Autodesk Inventor part; units mm, degrees
ref_plane "YZ Plane" through (0, 0, 0) normal (1, 0, 0) x (0, 1, 0)
ref_plane "XZ Plane" through (0, 0, 0) normal (0, 1, 0) x (-1, 0, 0)
ref_plane "XY Plane" through (0, 0, 0) normal (0, 0, 1) x (1, 0, 0)
sketch "Sketch1" plane through (0, 0, 0) normal (0, 0, 1) x (1, 0, 0)
  line L0 (0, 0) -> (3.175, 0)
  line L1 (3.175, 0) -> (3.175, 38.1)
  line L2 (3.175, 38.1) -> (0, 38.1)
  line L3 (0, 38.1) -> (0, 0)
  line L4 (0, 0) -> (38.1, 0)
  line L5 (38.1, 0) -> (38.1, 3.175)
  line L6 (38.1, 3.175) -> (0, 3.175)
  line L7 (0, 3.175) -> (0, 0)
  line L8 (38.1, 0) -> (34.925, 0)
  line L9 (34.925, 0) -> (34.925, 38.1)
  line L10 (34.925, 38.1) -> (38.1, 38.1)
  line L11 (38.1, 38.1) -> (38.1, 0)
  dimension "d0" = 3.175
  dimension "d1" = 38.1
  dimension "d2" = 38.1
  dimension "d3" = 3.175
  dimension "d4" = 3.175
  dimension "d5" = 38.1
extrude "Extrusion1" add sketch "Sketch1" along normal blind 101.6
sketch "Sketch2" plane through (38.1, 0, 0) normal (1, 0, 0) x (0, 0, -1)
  line L0 (-101.6, 3.175) -> (0, 3.175)
  line L1 (0, 0) -> (0, 38.1)
  point P0 (-7.9375, 9.525)
  dimension "d8" = 6.35
  dimension "d9" = 7.9375
hole "Hole1" at (38.1, 9.525, 7.9375) direction (-1, 0, 0) diameter 6.35 end through all
sketch "Sketch3" plane through (38.1, 0, 0) normal (1, 0, 0) x (0, 0, -1)
  line L0 (0, 38.1) -> (-101.6, 38.1)
  line L1 (0, 0) -> (0, 38.1)
  point P0 (-22.225, 31.75)
  dimension "d17" = 6.35
  dimension "d18" = 22.225
hole "Hole2" at (38.1, 31.75, 22.225) direction (-1, 0, 0) diameter 6.35 end through all
ref_plane "Work Plane1" through (19.05, 3.175, 0) normal (-1, 0, 0) x (0, 0, 1)
fillet "Fillet1" radius 12.7 1 edges at (19.05, 0, 0)
sketch "Sketch4" plane through (0, 0, 101.6) normal (-1, 0, 0) x (0, 0, 1)
  line L0 (-78.4449, 41.9138) -> (31.1063, -12.1864)
  line L1 (31.1063, -12.1864) -> (58.2522, 42.7832)
  line L2 (58.2522, 42.7832) -> (-51.299, 96.8833)
  line L3 (-51.299, 96.8833) -> (-78.4449, 41.9138)
  arc A0 (-101.6, 12.7) -> (-88.9, 0) centre (-88.9, 12.7) ccw
  line L4 (-88.9, 0) -> (0, 0)
  line L5 (0, 38.1) -> (0, 0)
  line L6 (-101.6, 38.1) -> (0, 38.1)
  line L7 (-101.6, 38.1) -> (-101.6, 12.7)
  circle A1 centre (-79.375, 31.75) radius 3.175
  circle A2 centre (-93.6625, 9.525) radius 3.175
  line L8 (-97.3003, 3.175) -> (0, 3.175)
  point P0 (-101.6, 0)
  dimension "d27" = 9.525
  dimension "d28" = 6.35
extrude "Extrusion2" cut sketch "Sketch4" against normal through all contours L5 L6 L0 L3 L2 L1 | L0 L6 L5
fillet "Fillet2" radius 15.875 2 edges at (1.5875, 38.1, 0) (36.5125, 38.1, 0)
sketch "Sketch5" plane through (0, 0, 101.6) normal (0, -1, 0) x (1, 0, 0)
  line L0 (0, -88.9) -> (0, 0)
  point P0 (0, -101.6)
  point P1 (19.05, -25.4)
  dimension "d32" = 19.05
  dimension "d40" = 76.2
hole "Hole3" at (19.05, 0, 76.2) direction (0, 1, 0) diameter 6.35 end through all
sketch "Sketch6" plane through (0, 0, 101.6) normal (0, -1, 0) x (1, 0, 0)
  circle A0 centre (19.05, -25.4) radius 3.175
  circle A1 centre (19.05, -25.4) radius 3.175
  line L0 (38.1, -88.9) -> (0, -88.9)
  line L1 (38.1, -88.9) -> (38.1, 0)
  line L2 (0, 0) -> (38.1, 0)
  line L3 (0, -88.9) -> (0, 0)
  line L4 (-11.1164, -15.875) -> (47.1756, -15.875)
  line L5 (47.1756, -15.875) -> (47.1756, 8.1032)
  line L6 (47.1756, 8.1032) -> (-11.1164, 8.1032)
  line L7 (-11.1164, 8.1032) -> (-11.1164, -15.875)
  point P0 (0, -101.6)
  dimension "d41" = 9.525
  dimension "d42" = 6.35
extrude "Extrusion3" cut sketch "Sketch6" against normal through all contours L4 L3 L2 L1 | L1 L2 L3 L4 L7 L6 L5
fillet "Fillet3" radius 19.05 2 edges at (0, 5.5073, 85.725) (38.1, 5.5073, 85.725)
sketch "Sketch7" plane through (0, 0, 12.7) normal (0, -1, 0) x (1, 0, 0)
  circle A0 centre (19.05, 63.5) radius 3.175
  line L0 (19.05, 63.5) -> (19.05, 60.325) construction
  line L1 (15.875, 63.5) -> (15.875, 60.325)
  line L2 (22.225, 60.325) -> (22.225, 63.5)
  arc A1 (22.225, 63.5) -> (15.875, 63.5) centre (19.05, 63.5) ccw
  arc A2 (15.875, 60.325) -> (22.225, 60.325) centre (19.05, 60.325) ccw
  point P0 (0, -12.7)
  point P1 (19.05, 61.9125)
  dimension "d46" = 3.175
extrude "Extrusion4" cut sketch "Sketch7" against normal blind 25.4 contours L2 A2 L1 A0
properties part number "CAR_048_NewCarouselTensioner1.5UChannel" material "Aluminum 6061"
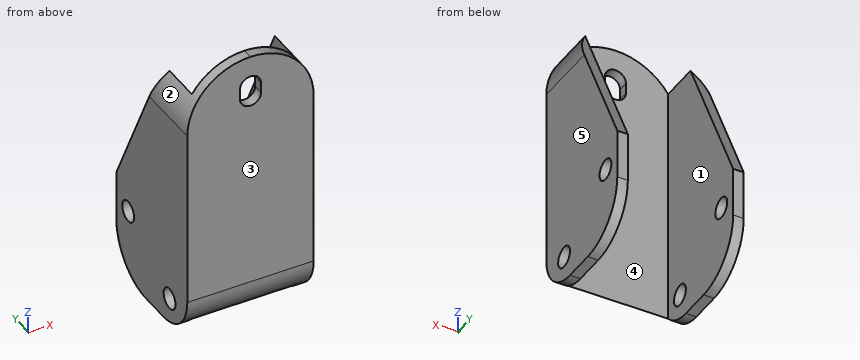
Part model, mm, in its own coordinate system. Face numbers are marked on the shaded views. A direction names the side the tool comes from. Give positions to 0.01 mm unless a question says otherwise; leave off trailing zeros. Write each loop counter-clockwise with the first axis right and the second up, starting at its lowest first coordinate (ties: lowest second). Pieces come first, ordered by that corner, then holes. Notation, with made-up numbers: (62.25, -16.5) -> (87.25, -16.5) arc R23 cw to (87.25, 17.5) -> close; hole circle Ø4 at (62, 78.5). An arc over 180 degrees is marked (long way). Put each result on its own line as item: value. Start each with the question number.
Item 1: Wall check: L1, parallel to X at y = 20.5, z = 54 (3 decimals); L2, parallel to Y at x = 13, z = 60 (3 decimals); L3, parallel to Z at x = 16.5, y = 2.5. Give the ranges that are in metal, low to high. Write a range as [from, to].
Item 2: Which spindle directions (+Z, -Z, +X, -X, +Y, -Y) get a long thin tool onto all of the face, cutting with end or side? Do the marked faces 4 and 5. Say none if no direction does.
Item 3: Pin check, flat tips, straight feed: pin 1 Ø3 at (x, z) = (26, 69.5) entering from +Y (3 decimals); pin 2 Ø6 at (y, z) = (29.5, 60) entering from -X; pin 3 Ø2.5 at (y, z) = (1.5, 75) entering from -X; pin 4 Ø1 at (x, z) = (17.5, 9) entering from -Y. Stop position of each tip, or through.
Item 4: Pull direction X, two halves, no side cores. Call the marked faces 1, 2 and 3: pulls with the +X half, pulls with the -X half, needs draft (parallel to the pull), parting line crosses it, or undercut.
Item 5: Cut at A-A (y = 16.5). List the corners of the cut face in (x, z) (3 decimals), then the cut area to 3 significant figures.
Item 6: Cut at D-D (x = 14). List the corners of the cut face in (y, z) (3 decimals).
Item 7: Cut at B-B (y = 31.75). List the corners of the cut face in (x, z) (3 decimals).
Item 8: Cut at C-C (z = 65.5). List the corners of the cut face in (x, y) (3 decimals), then the cut area to 3 significant figures.
Answer list:
1. L1: x = [0, 3.175], [34.925, 38.1]
1. L2: y = [0, 3.175]
1. L3: z = [5.13, 71.13], [78.09, 85.55]
2. face 4: +Z, -Z, +Y
2. face 5: +Z, -Z, +X, +Y, -Y
3. pin 1: stops at y = 3.175
3. pin 2: passes through
3. pin 3: stops at x = 1.36
3. pin 4: stops at y = 0.41
4. face 1: undercut
4. face 2: pulls with the -X half
4. face 3: needs draft
5. outline: (0, 0) -> (3.175, 0) -> (3.175, 74.617) -> (1.735, 74.617) arc R19.05 ccw to (0, 66.675) -> close; (34.925, 0) -> (38.1, 0) -> (38.1, 66.675) arc R19.05 ccw to (36.365, 74.617) -> (34.925, 74.617) -> close
5. area: 465 mm2
6. outline: (0, 12.7) arc R12.7 ccw to (3.175, 4.3) -> (3.175, 85.043) -> (0, 85.043) -> close
7. outline: (0, 3.175) -> (3.175, 3.175) -> (3.175, 19.05) -> (0, 19.05) -> close; (0, 25.4) -> (3.175, 25.4) -> (3.175, 43.736) -> (0, 43.736) -> close; (34.925, 3.175) -> (38.1, 3.175) -> (38.1, 19.05) -> (34.925, 19.05) -> close; (34.925, 25.4) -> (38.1, 25.4) -> (38.1, 43.736) -> (34.925, 43.736) -> close
8. outline: (0, 0) -> (38.1, 0) -> (38.1, 21.002) -> (34.925, 21.002) -> (34.925, 3.175) -> (3.175, 3.175) -> (3.175, 21.002) -> (0, 21.002) -> close
8. area: 234 mm2
